Source: CAD feature listing. Evaluate the final solid. Frame: model axes, mm. A direction names the side the tool comes from. Coordinates: 2 decimals unless noted, no trailing zeros. Loops run counter-clockwise (first coordinate to the right, second up) from the corner with the lowest first, then second, coordinate; pieces in that order, holes last. Notation, with made-up numbers: (79.5, -13) -> (133.5, -13) arc R21 cw to (133.5, 8) -> close; hole circle Ø1 at (21.25, -22). An arc over 180 degrees is marked (long way). Answer as a JSON object with one key per item and string values. Group by question number.
from build123d import *

# Parameters (mm, degrees)
ESTRUSIONE_ESTRUSIONE1_DEPTH = 2.5
CORTAR_EXTRUIR4_DEPTH        = 10
CROQUIS2_R                   = 2.05
CORTAR_EXTRUIR5_DEPTH        = 6
CUT_EXTRUDE1_REACH           = 7
SKETCH3_W                    = 4.1
SKETCH3_H                    = 30
CUT_EXTRUDE2_REACH           = 7
SKETCH4_R                    = 2.05


with BuildPart() as part:
    # Schizzo1 → Estrusione-Estrusione1 (new body, symmetric)
    with BuildSketch(Plane(origin=(0, 0, 0), x_dir=(1, 0, 0), z_dir=(0, 1, 0))):
        with BuildLine():
            Line((-25, 37.416573868), (-25, 26.25))
            Line((-25, 26.25), (25, 26.25))
            Line((25, 26.25), (25, 37.416573868))
            ThreePointArc((25, 37.416573868), (45, 0), (25, -37.416573868))
            Line((25, -37.416573868), (25, -26.25))
            Line((25, -26.25), (-25, -26.25))
            Line((-25, -26.25), (-25, -37.416573868))
            ThreePointArc((-25, -37.416573868), (-45, 0), (-25, 37.416573868))
        make_face()
    extrude(amount=ESTRUSIONE_ESTRUSIONE1_DEPTH, both=True)

    # Croquis1 → Cortar-Extruir4 (cut)
    with BuildSketch(Plane.XZ.offset(2.5)):
        Polygon((-8.5, 26.25), (-11.5, 26.25), (-11.5, 18.25), (-12.75, 18.25), (-12.75, 15.25), (-11.5, 15.25), (-11.5, 12.25), (-8.5, 12.25), (-8.5, 15.25), (-7.25, 15.25), (-7.25, 18.25), (-8.5, 18.25), align=None)
        Polygon((11.5, 26.25), (8.5, 26.25), (8.5, 18.25), (7.25, 18.25), (7.25, 15.25), (8.5, 15.25), (8.5, 12.25), (11.5, 12.25), (11.5, 15.25), (12.75, 15.25), (12.75, 18.25), (11.5, 18.25), align=None)
        Polygon((8.5, -12.25), (8.5, -15.25), (7.25, -15.25), (7.25, -18.25), (8.5, -18.25), (8.5, -26.25), (11.5, -26.25), (11.5, -18.25), (12.75, -18.25), (12.75, -15.25), (11.5, -15.25), (11.5, -12.25), align=None)
        Polygon((-11.5, -12.25), (-11.5, -15.25), (-12.75, -15.25), (-12.75, -18.25), (-11.5, -18.25), (-11.5, -26.25), (-8.5, -26.25), (-8.5, -18.25), (-7.25, -18.25), (-7.25, -15.25), (-8.5, -15.25), (-8.5, -12.25), align=None)
    extrude(amount=-CORTAR_EXTRUIR4_DEPTH, mode=Mode.SUBTRACT)

    # Croquis2 → Cortar-Extruir5 (cut, through all)
    with BuildSketch(Plane(origin=(0, 2.5, 0), x_dir=(1, 0, 0), z_dir=(0, 1, 0))):
        with Locations((0, 20.25)):
            Circle(CROQUIS2_R)
        with Locations((0, -20.25)):
            Circle(CROQUIS2_R)
    extrude(amount=-CORTAR_EXTRUIR5_DEPTH, mode=Mode.SUBTRACT)

    # Sketch3 → Cut-Extrude1 (cut, up to next)
    with BuildSketch(Plane(origin=(0, 2.5, 0), x_dir=(1, 0, 0), z_dir=(0, 1, 0)), mode=Mode.PRIVATE) as cut_extrude1_sk1:
        with Locations((-20.45, 0)):
            Rectangle(SKETCH3_W, SKETCH3_H)
    cut_extrude1_tool1 = extrude(cut_extrude1_sk1.sketch, amount=-CUT_EXTRUDE1_REACH, mode=Mode.PRIVATE) & part.part
    add(cut_extrude1_tool1.solids().sort_by_distance((-20.45, 2.5, 0))[0], mode=Mode.SUBTRACT)

    # Sketch4 → Cut-Extrude2 (cut, up to next)
    with BuildSketch(Plane(origin=(0, 2.5, 0), x_dir=(1, 0, 0), z_dir=(0, 1, 0)), mode=Mode.PRIVATE) as cut_extrude2_sk1:
        with Locations((-25, 26.25)):
            Circle(SKETCH4_R)
    cut_extrude2_tool1 = extrude(cut_extrude2_sk1.sketch, amount=-CUT_EXTRUDE2_REACH, mode=Mode.PRIVATE) & part.part
    add(cut_extrude2_tool1.solids().sort_by_distance((-25, 2.5, -26.25))[0], mode=Mode.SUBTRACT)
    # Sketch4 → Cut-Extrude2 (cut, up to next)
    with BuildSketch(Plane(origin=(0, 2.5, 0), x_dir=(1, 0, 0), z_dir=(0, 1, 0)), mode=Mode.PRIVATE) as cut_extrude2_sk2:
        with Locations((-25, -26.25)):
            Circle(SKETCH4_R)
    cut_extrude2_tool2 = extrude(cut_extrude2_sk2.sketch, amount=-CUT_EXTRUDE2_REACH, mode=Mode.PRIVATE) & part.part
    add(cut_extrude2_tool2.solids().sort_by_distance((-25, 2.5, 26.25))[0], mode=Mode.SUBTRACT)
    # Sketch4 → Cut-Extrude2 (cut, up to next)
    with BuildSketch(Plane(origin=(0, 2.5, 0), x_dir=(1, 0, 0), z_dir=(0, 1, 0)), mode=Mode.PRIVATE) as cut_extrude2_sk3:
        with Locations((25, -26.25)):
            Circle(SKETCH4_R)
    cut_extrude2_tool3 = extrude(cut_extrude2_sk3.sketch, amount=-CUT_EXTRUDE2_REACH, mode=Mode.PRIVATE) & part.part
    add(cut_extrude2_tool3.solids().sort_by_distance((25, 2.5, 26.25))[0], mode=Mode.SUBTRACT)
    # Sketch4 → Cut-Extrude2 (cut, up to next)
    with BuildSketch(Plane(origin=(0, 2.5, 0), x_dir=(1, 0, 0), z_dir=(0, 1, 0)), mode=Mode.PRIVATE) as cut_extrude2_sk4:
        with Locations((25, 26.25)):
            Circle(SKETCH4_R)
    cut_extrude2_tool4 = extrude(cut_extrude2_sk4.sketch, amount=-CUT_EXTRUDE2_REACH, mode=Mode.PRIVATE) & part.part
    add(cut_extrude2_tool4.solids().sort_by_distance((25, 2.5, -26.25))[0], mode=Mode.SUBTRACT)


solid = part.part
1. Mould query, pull axis X, two halves, no side actions, for faces 1 (the face through (1, -2.5, -1)), 2 (the face through (-1.511, 0.035, 18.865)). Classes: pulls with the +X half, pulls with the -X half, needs draft (parallel to the pull), parting line crosses it, or undercut.
2. Section query B-B on z = 4.5. Return loops of the section in (x, y), then the cut area to 3 significant figures.
3. Section query A-A on x = 0. Return loops of the section in (y, z).
4. Section query D-D on y = -1.7. State how many separate pieces and enclosed holes the cut face has, then the cut area to 3 significant figures.
5. Pin query (flat end, axial travel): pin 1 Ø2.5 at (y, z) = (0, 13) entering from +X; pin 2 Ø1.5 at (y, z) = (0.5, -32) entering from -X; pin 3 Ø0.6 at (x, y) = (12, -0.5) entering from +Z. Return the tip coordinate at first contact, or that it passes through.
6. Ray query, L1, parallel to Z at x = 0, y = -0.35; L2, parallel to X at y = 1, z = 22; L3, parallel to Z at x = 1.5, y = 1.5. Return the intervals inside material, ascending.
7. Reachability of faces 3 (the face through (10, 0, 12.25)), 4 (the face through (10, 0, -12.25)), 5 (the face through (-22.5, 0, 0)) from +Z, -Z, +X, -X, +Y, -Y: full face, straight path, thin tool, end or side. Return the list, or none.
8. Section query C-C on z = 20.25. Return loops of the section in (x, y), then the cut area to 3 significant figures.
Solved:
{
 "1": {"face 1": "needs draft", "face 2": "undercut"},
 "2": {"outline": "(-44.77, -2.5) -> (-22.5, -2.5) -> (-22.5, 2.5) -> (-44.77, 2.5) -> close; (-18.4, -2.5) -> (44.77, -2.5) -> (44.77, 2.5) -> (-18.4, 2.5) -> close", "area": "427 mm^2"},
 "3": {"outline": "(-2.5, -26.25) -> (2.5, -26.25) -> (2.5, -22.3) -> (-2.5, -22.3) -> close; (-2.5, -18.2) -> (2.5, -18.2) -> (2.5, 18.2) -> (-2.5, 18.2) -> close; (-2.5, 22.3) -> (2.5, 22.3) -> (2.5, 26.25) -> (-2.5, 26.25) -> close"},
 "4": {"separate pieces": "1", "enclosed holes": "3", "area": "4,340 mm^2"},
 "5": {"pin 1": "x = 43.44", "pin 2": "x = -32.38", "pin 3": "z = 26.25"},
 "6": {"L1": "-26.25 to -22.3, -18.2 to 18.2, 22.3 to 26.25", "L2": "-39.26 to -11.5, -8.5 to -1.07, 1.07 to 8.5, 11.5 to 39.26", "L3": "-26.25 to -21.65, -18.85 to 18.85, 21.65 to 26.25"},
 "7": {"face 3": "+Z, +Y, -Y", "face 4": "-Z, +Y, -Y", "face 5": "+Y, -Y"},
 "8": {"outline": "(-40.19, -2.5) -> (-11.5, -2.5) -> (-11.5, 2.5) -> (-40.19, 2.5) -> close; (-8.5, -2.5) -> (-2.05, -2.5) -> (-2.05, 2.5) -> (-8.5, 2.5) -> close; (2.05, -2.5) -> (8.5, -2.5) -> (8.5, 2.5) -> (2.05, 2.5) -> close; (11.5, -2.5) -> (40.19, -2.5) -> (40.19, 2.5) -> (11.5, 2.5) -> close", "area": "351 mm^2"}
}
